The listing builds one solid part. Answer for the finished solid, in the listing's coordinates (mm). A direction names the side the tool comes from. Coordinates: 2 decimals unless noted, no trailing zeros. Order: outer loops, then holes, each group sorted by start corner. A loop starts at its lowest first (then second) coordinate and runs counter-clockwise, first axis right, second up. Notation, with made-up numbers: (52, 41) -> (92, 41) arc R19 ccw to (92, 75) -> close; hole circle Ø6 at (-28.5, -39.5). An arc over 180 degrees is marked (long way). Return JSON: item names as keys, results as strings.
from build123d import *

# Parameters (mm, degrees)
SKETCH1_R           = 1.27
BOSS_EXTRUDE1_DEPTH = 119.9642
SKETCH3_R           = 0.762
BOSS_EXTRUDE2_DEPTH = 3.175
CHAMFER1_SIZE       = 0.508


with BuildPart() as part:
    # Sketch1 → Boss-Extrude1 (new body)
    with BuildSketch(Plane.XY):
        with Locations(Location((0, 0, 0), (0, 0, 180))):
            Circle(SKETCH1_R)
    extrude(amount=BOSS_EXTRUDE1_DEPTH)

    # Sketch3 → Boss-Extrude2 (add)
    with BuildSketch(Plane.XY.offset(119.9642)):
        Circle(SKETCH3_R)
    extrude(amount=BOSS_EXTRUDE2_DEPTH)

    # Chamfer1
    chamfer1_edges = [part.edges().sort_by_distance(p)[0] for p in [
        (-0.762, 0, 123.1392),
    ]]
    chamfer(chamfer1_edges, length=CHAMFER1_SIZE)


solid = part.part
1. Consider line 1 (Z direction, x = 1.05, y = -0.4); line 2 (Y direction, x = 1, z = 62); line 3 (X direction, y = 0.1, z = 76.5). Determine where each line is inside the solid, lowest interval first. Write a range as from..to.
Answer block:
{"line 1": "z = 0..119.96", "line 2": "y = -0.78..0.78", "line 3": "x = -1.27..1.27"}
2. The part is cut by section A-A on z = 32.5. Give the vertices of the cut face in (x, y).
Answer block:
{"outline": "circle Ø2.54 at (0, 0)"}
3. For faces 1 (the face through (0, 1, 119.964)), 2 (the face through (0.17, -1.26, 59.14)), determine the directions among +Z, -Z, +X, -X, +Y, -Y from which every point of the face is accessible in a straight line to the end or side of a thin tool.
Answer block:
{"face 1": "+Z", "face 2": "+Z, -Z"}
